Input: part model. Units: mm. Frame: model coordinates. A direction names the side the tool comes from. Give positions to 0.01 mm unless a question says otherwise; leave off trailing zeros. Loops run counter-clockwise (first coordinate to the right, second up) from the corner with the lowest first, then second, coordinate; pieces in that order, holes last. Notation, with made-up numbers: (60, -2.5) -> (85, -2.5) arc R19 cw to (85, 20.5) -> close; hole circle Ø2 at (56, 5.25). An arc over 180 degrees is marked (long way). One line per question, with ' | ' between items.
from build123d import *

# Parameters (mm, degrees)
SKETCH1_R          = 3.175
EXTRUDE1_DEPTH     = 38.1
CHAMFER3_SIZE      = 0.9525
SKETCH6_R          = 4.7625
EXTRUDE2_DEPTH     = 6.35
CUT_EXTRUDE1_DEPTH = 3.571875
CHAMFER1_SIZE      = 0.47625
CHAMFER2_SIZE      = 0.238125


with BuildPart() as part:
    # Sketch1 → Extrude1 (new body)
    with BuildSketch(Plane.XY):
        Circle(SKETCH1_R)
    extrude(amount=-EXTRUDE1_DEPTH)

    # Chamfer3
    chamfer3_edges = [part.edges().sort_by_distance(p)[0] for p in [
        (-3.175, 0, 0),
    ]]
    chamfer(chamfer3_edges, length=CHAMFER3_SIZE)

    # Sketch6 → Extrude2 (add)
    with BuildSketch(Plane(origin=(0, 0, -38.1), x_dir=(-1, 0, 0), z_dir=(0, 0, -1))):
        Circle(SKETCH6_R)
    extrude(amount=EXTRUDE2_DEPTH)

    # Sketch7 → Cut-Extrude1 (cut)
    with BuildSketch(Plane(origin=(0, 0, -44.45), x_dir=(-1, 0, 0), z_dir=(0, 0, -1))):
        Polygon((0, 2.749630657), (-2.38125, 1.374815329), (-2.38125, -1.374815329), (0, -2.749630657), (2.38125, -1.374815329), (2.38125, 1.374815329), align=None)
    extrude(amount=-CUT_EXTRUDE1_DEPTH, mode=Mode.SUBTRACT)

    # Cut-Extrude2 cone 1 section (through the dimple's axis) → Cut-Extrude2 (revolve, cut)
    with BuildSketch(Plane(origin=(0, 0, -44.45), x_dir=(0, 1, 0), z_dir=(1, 0, 0))):
        Polygon((0, 0), (2.749630657, 0), (0, 2.749630657), align=None)
    revolve(axis=Axis((0, 0, -44.45), (0, 0, 1)), mode=Mode.SUBTRACT)

    # Chamfer1
    chamfer1_edges = [part.edges().sort_by_distance(p)[0] for p in [
        (4.7625, 0, -44.45),
    ]]
    chamfer(chamfer1_edges, length=CHAMFER1_SIZE)

    # Chamfer2
    chamfer2_edges = [part.edges().sort_by_distance(p)[0] for p in [
        (4.7625, 0, -38.1),
    ]]
    chamfer(chamfer2_edges, length=CHAMFER2_SIZE)


solid = part.part
1. Pin query (flat end, axial travel): P1, Ø2.5, axis at x = -0.5, y = 0, coming from the -Z side; P2, Ø3, axis at x = -1.5, y = -3.5, coming from the +Z side; P3, Ø5, axis at x = 1.5, y = 3, coming from the +Z side; P4, Ø3, axis at y = -3.5, z = -20, coming from the -X side. Return the tip coordinate at first contact, or that it passes through.
Determined:
P1: stops at z = -40.88 | P2: stops at z = -0.09 | P3: stops at z = 0 | P4: stops at x = -2.47
2. Pull-direction query (Y, two-part tool) for faces 1 (the flat face through (-2, -3, -38.1)), 2 (the flat face through (-2.381, 0, -43)), 3 (the cylindrical face through (-0.69, -3.1, -19.27)), 4 (the flat face through (-1.174, -2.072, -42.689)); classes: pulls with the +Y half, pulls with the -Y half, needs draft (parallel to the pull), parting line crosses it, or undercut.
Determined:
face 1: needs draft | face 2: undercut | face 3: parting line crosses it | face 4: undercut
3. Section query B-B (z = -3.5). Output: boundary loops of the cut face in (x, y) (3 decimals), then the cut area to 3 significant figures.
Determined:
outline: circle Ø6.35 at (0, 0) | area: 31.7 mm2
4. Reachability of faces 5 (the flat face through (1.21, -2.05, -42.69)), 6 (the flat face through (0, -3, -44.45)) from +Z, -Z, +X, -X, +Y, -Y: full face, straight path, thin tool, end or side. Return the list, or none.
Determined:
face 5: -Z | face 6: -Z, +X, -X, +Y, -Y
5. Ray query, line 1 along Z through (x, y) = (-0.25, 1); line 2 along Z through (x, y) = (0.75, 3.5); line 3 along Y through (x, z) = (-0.25, -21). Return the intervals inside material, ascending. Write a range as from..to.
Determined:
line 1: z = -40.88..0 | line 2: z = -44.45..-38.1 | line 3: y = -3.17..3.17
